Check sheet for the modelled part. Datum: model origin and axes. Units: mm. Face numbers are marked on the shaded views. A direction names the side the tool comes from. Coordinates: 2 decimals unless noted, no trailing zeros. Write each loop counter-clockwise with the first axis right and the second up, starting at its lowest first coordinate (ties: lowest second). Pieces come first, ordered by that corner, then holes. Notation, with made-up numbers: M 26.25,47 L 37.25,47 A20 ccw 37.25,71 Z; hole C -38,20.25 d8. An arc over 180 degrees is marked long. Answer as CSV lines item,"result". Start each with the question number.
Q1. Sectioned sample at B-B, the plane y = 10. Record the cut outline in (x, z), then the cut area to 3 significant figures.
Q2. Sectioned sample at C-C, the plane x = 0. Record the cut outline in (y, z), then the cut area to 3 significant figures.
Q3. Thickness scan on line 1 along Y through (x, z) = (-19.5, 0.5); line 2 along X through (y, z) = (12, -10.5); line 3 along X through (y, z) = (11, -5). Record the ranges inside material, lowest first. Write a range as from..to.
Q4. Depth check by flat-ended pin: pin 1 Ø8 at (y, z) = (12, -7.5) entering from -X; pin 2 Ø8 at (x, y) = (5, 6.5) entering from -Z; pin 3 Ø10 at (x, y) = (-14.5, -12) entering from +Z. Enter the tip coordinate at first touch or a pass-through.
Q5. Access from +Z, -Z, +X, -X, +Y, -Y to the whole of each face (thin tool, end or side, straight path). Record for the marked faces 1, 2 and 3.
Q6. Sectioned sample at D-D, the plane y = 2. Record the cut outline in (x, z).
Q7. Mould release check, pull along Z, two halves, no side actions. Record for the marked faces 4, 5 and 6: pulls with the +Z half, pulls with the -Z half, needs draft (parallel to the pull), parting line crosses it, or undercut.
Q8. Sectioned sample at A-A, the plane z = 0. Record the cut outline in (x, y).
from build123d import *

# Parameters (mm, degrees)
F0_R     = 21.59
F1_DEPTH = 15.24
F2_W     = 41.967688
F2_H     = 10.16
F3_DEPTH = 10.16
F4_W     = 10.16
F4_H     = 41.967688
F5_DEPTH = 10.16


with BuildPart() as f1:
    # F0 (on Front) → F1 (new body, symmetric)
    with BuildSketch(Plane.XZ):
        Circle(F0_R)
    extrude(amount=F1_DEPTH, both=True)

    # F2 (on face) → F3 (cut)
    with BuildSketch(Plane.XZ.offset(15.24)):
        Rectangle(F2_W, F2_H)
        with BuildLine():
            ThreePointArc((-20.983844, 5.08), (-21.59, 0), (-20.983844, -5.08))
            Line((-20.983844, -5.08), (-20.983844, 5.08))
        make_face()
        with BuildLine():
            Line((20.983844, 5.08), (20.983844, -5.08))
            ThreePointArc((20.983844, -5.08), (21.437925, -2.558018), (21.59, 0))
            ThreePointArc((21.59, 0), (21.437925, 2.558018), (20.983844, 5.08))
        make_face()
    extrude(amount=-F3_DEPTH, mode=Mode.SUBTRACT)

    # F4 (on face) → F5 (cut)
    with BuildSketch(Plane(origin=(0, 15.24, 0), x_dir=(-1, 0, 0), z_dir=(0, 1, 0))):
        with BuildLine():
            ThreePointArc((5.08, 20.983844), (0, 21.59), (-5.08, 20.983844))
            Line((-5.08, 20.983844), (5.08, 20.983844))
        make_face()
        Rectangle(F4_W, F4_H)
        with BuildLine():
            Line((5.08, -20.983844), (-5.08, -20.983844))
            ThreePointArc((-5.08, -20.983844), (0, -21.59), (5.08, -20.983844))
        make_face()
    extrude(amount=-F5_DEPTH, mode=Mode.SUBTRACT)


solid = f1.part
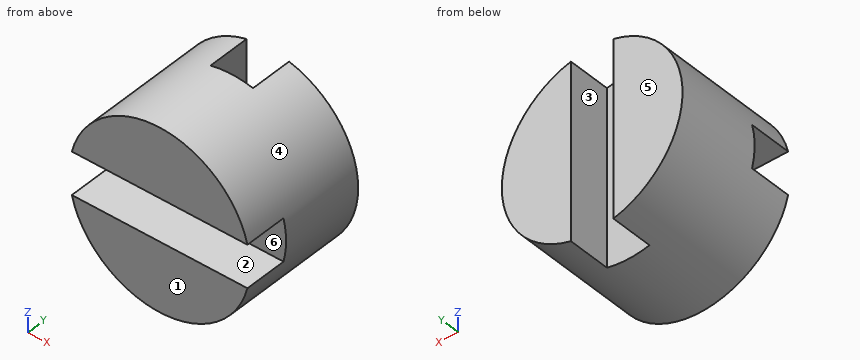
Output:
1,outline,"M -5.08,-20.98 L -5.08,20.98 A21.59 ccw Z; M 5.08,-20.98 A21.59 ccw 5.08,20.98 Z"
1,area,"1,030 mm^2"
2,outline,"M -15.24,-21.59 L 5.08,-21.59 L 5.08,21.59 L -15.24,21.59 L -15.24,5.08 L -5.08,5.08 L -5.08,-5.08 L -15.24,-5.08 Z"
2,area,"774 mm^2"
3,line 1,"y = -5.08..15.24"
3,line 2,"x = -18.86..-5.08, 5.08..18.86"
3,line 3,"x = -21..-5.08, 5.08..21"
4,pin 1,"stops at x = -21.3"
4,pin 2,"stops at z = -21.55"
4,pin 3,"stops at z = 19.39"
5,face 1,"+Z, -Z, +X, -X, -Y"
5,face 2,"+X, -X, -Y"
5,face 3,"+Z, -Z, +Y"
6,outline,"C 0,0 d43.18"
7,face 4,"parting line crosses it"
7,face 5,"needs draft"
7,face 6,"undercut"
8,outline,"M -21.59,-5.08 L 21.59,-5.08 L 21.59,15.24 L 5.08,15.24 L 5.08,5.08 L -5.08,5.08 L -5.08,15.24 L -21.59,15.24 Z"
